Can you work these out from the drawing? Everything is in mm from the part's minimum corner. A direction names the side the tool comes from. Coordinates: 2 decimals unless noted, no trailing zeros. Write each loop counter-clockwise with the first axis right and the second up, starting at its lowest first coordinate (ties: lowest second). Pieces come first, ordered by that corner, then holes. Notation, with made-up numbers: (-2.75, 75.25) -> (33.25, 75.25) arc R15 ccw to (33.25, 93.25) -> close; hole circle Ø4 at (22.25, 17). An arc over 180 degrees is marked (long way). Use CSV: the item, a comma, the result in double quotes. Start each with the question number.
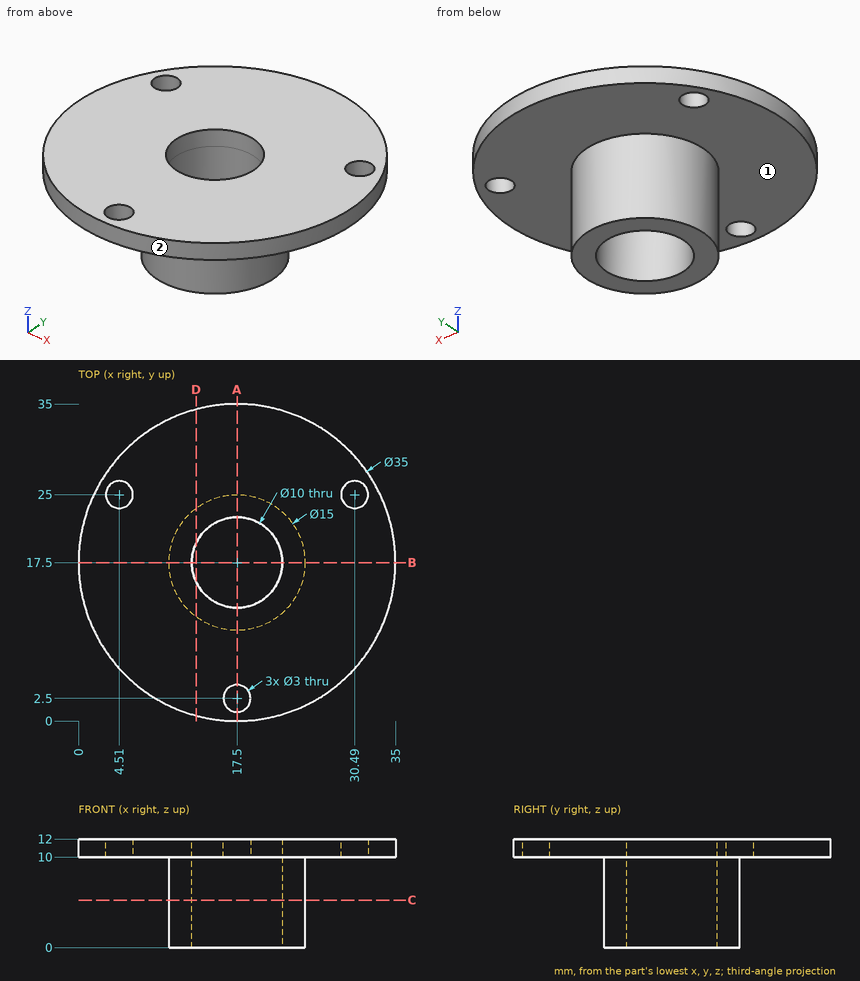
Item 1: If I drill on line 1 along Y through (x, z) = (17.5, 11.35); line 2 along Z through (x, y) = (21, 26.5); line 3 along X through (y, z) = (18, 8.5) (1 decimal), over which ranges is the centre line in solid material (lowest first)?
Item 2: I want a section at C-C on z = 5.25. Please give me the cut outline in (x, y).
Item 3: I want a section at B-B on y = 17.5. Please give me the cut outline in (x, z), then the cut area to 3 significant figures.
Item 4: I'm going to push flat-ended pins straight in: pin 1 (12 mm diameter, centred on x = 19, y = 22.5, fed in from -Z); pin 2 (1.5 mm diameter, centred on x = 23.5, y = 8.5, fed in from -Z); pin 3 (1.5 mm diameter, centred on y = 25, z = 3, fed in from +X); pin 4 (1.5 mm diameter, centred on y = 21, z = 7, fed in from -X). Where does each tip first touch, or does it pass through?
Item 5: I want a section at A-A on x = 17.5. Please give me the cut outline in (y, z).
Item 6: I want a section at D-D on x = 13. Please give me the cut outline in (y, z), then the cut area to 3 significant figures.
Item 7: Which directions (+Z, -Z, +X, -X, +Y, -Y) give clear straight access to the entire face, cutting with the end or side of a thin tool? Please do the marked faces 1 and 2.
Geometry says:
1,line 1,"0 to 1, 4 to 12.5, 22.5 to 35"
1,line 2,"10 to 12"
1,line 3,"10 to 12.5, 22.5 to 25"
2,outline,"circle Ø15 at (17.5, 17.5); hole circle Ø10 at (17.5, 17.5)"
3,outline,"(0, 10) -> (10, 10) -> (10, 0) -> (12.5, 0) -> (12.5, 12) -> (0, 12) -> close; (22.5, 0) -> (25, 0) -> (25, 10) -> (35, 10) -> (35, 12) -> (22.5, 12) -> close"
3,area,"100 mm2"
4,pin 1,"z = 0"
4,pin 2,"z = 10"
4,pin 3,"x = 20.77"
4,pin 4,"x = 10.52"
5,outline,"(0, 10) -> (1, 10) -> (1, 12) -> (0, 12) -> close; (4, 10) -> (10, 10) -> (10, 0) -> (12.5, 0) -> (12.5, 12) -> (4, 12) -> close; (22.5, 0) -> (25, 0) -> (25, 10) -> (35, 10) -> (35, 12) -> (22.5, 12) -> close"
6,outline,"(0.59, 10) -> (11.5, 10) -> (11.5, 0) -> (15.32, 0) -> (15.32, 12) -> (0.59, 12) -> close; (19.68, 0) -> (23.5, 0) -> (23.5, 10) -> (34.41, 10) -> (34.41, 12) -> (19.68, 12) -> close"
6,area,"135 mm2"
7,face 1,"-Z"
7,face 2,"+Z, -Z"
